```python
from build123d import *

# Parameters (mm, degrees)
EXTRUDE_THIN2_DEPTH     = 40
CUT_EXTRUDE1_DEPTH      = 45.791182168
CUT_EXTRUDE1_DEPTH_BACK = 45.791182168
SKETCH2_W               = 6
SKETCH2_H               = 10
SKETCH3_R               = 2.35
CUT_EXTRUDE2_DEPTH      = 10


with BuildPart() as part:
    # Sketch1 → Extrude-Thin2 (new body)
    with BuildSketch(Plane.XY):
        with BuildLine():
            Line((20, -1.5), (0, -1.5))
            ThreePointArc((0, -1.5), (-0.736574842, 1.306697173), (1.283307019, -0.776610002))
            Line((1.283307019, -0.776610002), (2.138845031, -1.294350004))
            ThreePointArc((2.138845031, -1.294350004), (-1.227624737, 2.177828622), (0, -2.5))
            Line((0, -2.5), (20, -2.5))
            Line((20, -2.5), (20, -1.5))
        make_face()
    extrude(amount=EXTRUDE_THIN2_DEPTH)

    # Sketch2 → Cut-Extrude1 (cut, two sides: drawn at the far end of the back side and taken through both)
    with BuildSketch(Plane(origin=(0, 0, 0), x_dir=(1, 0, 0), z_dir=(0, 1, 0)).offset(-CUT_EXTRUDE1_DEPTH_BACK)):
        with Locations((0.5, -15)):
            Rectangle(SKETCH2_W, SKETCH2_H)
        with Locations((0.5, -35)):
            Rectangle(SKETCH2_W, SKETCH2_H)
    extrude(amount=CUT_EXTRUDE1_DEPTH + CUT_EXTRUDE1_DEPTH_BACK, mode=Mode.SUBTRACT)

    # Sketch3 → Cut-Extrude2 (cut)
    with BuildSketch(Plane(origin=(0, 0, 0), x_dir=(1, 0, 0), z_dir=(0, 1, 0))):
        with Locations((14.25, -20)):
            Circle(SKETCH3_R)
        with Locations((11.25, -34.05)):
            Circle(SKETCH3_R)
        with Locations((11.25, -5.95)):
            Circle(SKETCH3_R)
    extrude(amount=-CUT_EXTRUDE2_DEPTH, mode=Mode.SUBTRACT)


solid = part.part
```
For this review, take the finished solid that the model builds, in its own axes (mm). A direction names the side the tool comes from. Coordinates: 2 decimals unless noted, no trailing zeros. Loops run counter-clockwise (first coordinate to the right, second up) from the corner with the lowest first, then second, coordinate; pieces in that order, holes last. Notation, with made-up numbers: (-31, -32.5) - (-5, -32.5) arc R28 cw to (-5, -8.5) - close; hole circle Ø5 at (-27.75, 41.5). An arc over 180 degrees is marked (long way). Use one line per item in the form item = value. Start each with the question number.
1) Take a section at D-D (z = 5.95). State the section outline as (x, y) points.
2) Take a section at B-B (y = 0). State the section outline as (x, z) points, plus the area to 3 significant figures.
3) Take a section at C-C (x = 14.25). State the section outline as (y, z) points.
4) Draft analysis for pull direction Z (two halves, no side actions). For faces 4 (the face through (6, -2, 0)), 5 (the face through (-1.15, 2.22, 4.93)), 6 (the face through (3.5, -2, 15)), state which applies: released by +Z, released by -Z, zero draft, split by the parting line, or undercut.
5) Take a section at A-A (x = 11.25). State the section outline as (y, z) points.
6) To check wall thickness, follow probe 1 along Z at (x, y) = (11.25, -2); probe 2 along X at (y, z) = (0, 3.5); probe 3 along Z at (x, y) = (0, -1.75). State the ranges of each line that lie inside material, in increasing order. Write a range as from..to.
7) For faces 1 (the face through (0, -2, 10)), 2 (the face through (0, -2, 30)), 3 (the face through (1.705, -1.032, 4.93)), list the 3-axis set-ups (+Z, -Z, +X, -X, +Y, -Y) from which the entire face can be reached by the end or side of a thin tool; tool diameter is ignored.
8) For pin 1 (6 mm diameter, centred on x = 11.25, z = 34.05, fed in from -Y); pin 2 (0.8 mm diameter, centred on y = -2, z = 17.5, fed in from -X); pin 3 (4 mm diameter, centred on x = 14.25, z = 20, fed in from -Y); pin 4 (2.5 mm diameter, centred on x = 0, y = -0.5, fed in from +Z), all flat-tipped, find the tip position at first contact; note any pin that passes through.
From the geometry:
q1.outline = (0, -2.5) - (8.9, -2.5) - (8.9, -1.5) - (0, -1.5) arc R1.5 cw (long way) to (1.28, -0.78) - (2.14, -1.29) arc R2.5 ccw (long way) to start; (13.6, -2.5) - (20, -2.5) - (20, -1.5) - (13.6, -1.5) - close
q2.outline = (-2.5, 0) - (-1.5, 0) - (-1.5, 10) - (-2.5, 10) - close; (-2.5, 20) - (-1.5, 20) - (-1.5, 30) - (-2.5, 30) - close; (1.5, 0) - (2.5, 0) - (2.5, 10) - (1.5, 10) - close; (1.5, 20) - (2.5, 20) - (2.5, 30) - (1.5, 30) - close
q2.area = 40.0 mm2
q3.outline = (-2.5, 0) - (-1.5, 0) - (-1.5, 17.65) - (-2.5, 17.65) - close; (-2.5, 22.35) - (-1.5, 22.35) - (-1.5, 40) - (-2.5, 40) - close
q4.face_4 = released by -Z
q4.face_5 = zero draft
q4.face_6 = undercut
q5.outline = (-2.5, 0) - (-1.5, 0) - (-1.5, 3.6) - (-2.5, 3.6) - close; (-2.5, 8.3) - (-1.5, 8.3) - (-1.5, 31.7) - (-2.5, 31.7) - close; (-2.5, 36.4) - (-1.5, 36.4) - (-1.5, 40) - (-2.5, 40) - close
q6.probe_1 = 0..3.6, 8.3..31.7, 36.4..40
q6.probe_2 = -2.5..-1.5, 1.5..2.5
q6.probe_3 = 0..10, 20..30
q7.face_1 = -X, +Y, -Y
q7.face_2 = +Z, -X, +Y, -Y
q7.face_3 = +Z, -Z
q8.pin_1 = -2.5
q8.pin_2 = 3.5
q8.pin_3 = through
q8.pin_4 = 30
